```python
from build123d import *

# Parameters (mm, degrees)
SKETCH1_W           = 48.26
SKETCH1_H           = 38.1
BOSS_EXTRUDE1_DEPTH = 6.35
SKETCH2_R           = 3.683
CUT_EXTRUDE1_DEPTH  = 4.318
SKETCH3_R           = 2.159
CUT_EXTRUDE2_DEPTH  = 4.318
SKETCH4_R           = 1.143
CUT_EXTRUDE3_DEPTH  = 9.398
LPATTERN1_COUNT     = 3
LPATTERN1_PITCH     = 19.05
CUT_EXTRUDE7_DEPTH  = 4.318
CUT_EXTRUDE8_DEPTH  = 10.16


with BuildPart() as part:
    # Sketch1 → Boss-Extrude1 (new body)
    with BuildSketch(Plane(origin=(0, 0, 0), x_dir=(1, 0, 0), z_dir=(0, 1, 0))):
        Rectangle(SKETCH1_W, SKETCH1_H)
    extrude(amount=-BOSS_EXTRUDE1_DEPTH)

    # Sketch2 → Cut-Extrude1 (cut)
    with BuildSketch(Plane(origin=(0, 0, 0), x_dir=(1, 0, 0), z_dir=(0, 1, 0))):
        with Locations((-13.97, 0)):
            Circle(SKETCH2_R)
    cut_extrude1 = extrude(amount=-CUT_EXTRUDE1_DEPTH, mode=Mode.SUBTRACT)

    # Sketch3 → Cut-Extrude2 (cut)
    with BuildSketch(Plane(origin=(0, -4.318, 0), x_dir=(1, 0, 0), z_dir=(0, 1, 0))):
        with Locations((-13.97, 0)):
            Circle(SKETCH3_R)
    cut_extrude2 = extrude(amount=-CUT_EXTRUDE2_DEPTH, mode=Mode.SUBTRACT)

    # Sketch4 → Cut-Extrude3 (cut)
    with BuildSketch(Plane(origin=(0, 0, 0), x_dir=(1, 0, 0), z_dir=(0, 1, 0))):
        with Locations((-19.05, 15.621)):
            Circle(SKETCH4_R)
        with Locations((-19.05, -15.621)):
            Circle(SKETCH4_R)
    cut_extrude3 = extrude(amount=-CUT_EXTRUDE3_DEPTH, mode=Mode.SUBTRACT)

    # LPattern1: Cut-Extrude3 ×3
    with Locations(*[(i * LPATTERN1_PITCH, 0, 0) for i in range(1, LPATTERN1_COUNT)]):
        add(cut_extrude3, mode=Mode.SUBTRACT)

    # Mirror1: Cut-Extrude1, Cut-Extrude2 across plane
    add(cut_extrude1.mirror(Plane(origin=(0, 0, 0), x_dir=(0, 0, 1), z_dir=(1, 0, 0))), mode=Mode.SUBTRACT)
    add(cut_extrude2.mirror(Plane(origin=(0, 0, 0), x_dir=(0, 0, 1), z_dir=(1, 0, 0))), mode=Mode.SUBTRACT)

    # Sketch6 → Cut-Extrude7 (cut)
    with BuildSketch(Plane(origin=(0, 0, 0), x_dir=(1, 0, 0), z_dir=(0, 1, 0))):
        with BuildLine():
            Line((-17.653, -8.89), (-17.653, 8.89))
            ThreePointArc((-17.653, 8.89), (-13.97, 12.573), (-10.287, 8.89))
            Line((-10.287, 8.89), (-10.287, -8.89))
            ThreePointArc((-10.287, -8.89), (-13.97, -12.573), (-17.653, -8.89))
        make_face()
    cut_extrude7 = extrude(amount=-CUT_EXTRUDE7_DEPTH, mode=Mode.SUBTRACT)

    # Sketch7 → Cut-Extrude8 (cut)
    with BuildSketch(Plane(origin=(0, -4.318, 0), x_dir=(1, 0, 0), z_dir=(0, 1, 0))):
        with BuildLine():
            Line((-16.129, -8.89), (-16.129, 8.89))
            ThreePointArc((-16.129, 8.89), (-13.97, 11.049), (-11.811, 8.89))
            Line((-11.811, 8.89), (-11.811, -8.89))
            ThreePointArc((-11.811, -8.89), (-13.97, -11.049), (-16.129, -8.89))
        make_face()
    cut_extrude8 = extrude(amount=-CUT_EXTRUDE8_DEPTH, mode=Mode.SUBTRACT)

    # Mirror2: Cut-Extrude7, Cut-Extrude8 across plane
    add(cut_extrude7.mirror(Plane(origin=(0, 0, 0), x_dir=(0, 0, 1), z_dir=(1, 0, 0))), mode=Mode.SUBTRACT)
    add(cut_extrude8.mirror(Plane(origin=(0, 0, 0), x_dir=(0, 0, 1), z_dir=(1, 0, 0))), mode=Mode.SUBTRACT)


solid = part.part
```
Here's how the part is built. I have some questions about the finished solid (model axes, mm). A direction names the side the tool comes from. Round coordinates to 2 decimals unless told otherwise and drop trailing zeros. Loops run counter-clockwise (first coordinate to the right, second up) from the corner with the lowest first, then second, coordinate; pieces in that order, holes last.
1. Will these pins go through, and if not, where does the flat tip stop? pin 1 (1.8 mm diameter, centred on x = 0, z = 15.621, fed in from -Y); pin 2 (3.5 mm diameter, centred on x = 19.05, z = -15.621, fed in from +Y).
Answers:
pin 1: passes through
pin 2: stops at y = 0
2. Thinking about a two-plate mould opening in Z: for faces 1 (the face through (-16.129, -5, 0)), 2 (the face through (24.13, -3, 0)), 3 (the face through (0, -3, 19.05)), which applies, released by +Z, released by -Z, zero draft, split by the parting line, or undercut?
Answers:
face 1: undercut
face 2: zero draft
face 3: released by +Z
3. Suppose I cut it at A-A, the plane z = 5. Please give me the cut outline in (x, y).
Answers:
outline: (-24.13, -6.35) - (-16.13, -6.35) - (-16.13, -4.32) - (-17.65, -4.32) - (-17.65, 0) - (-24.13, 0) - close; (-11.81, -6.35) - (11.81, -6.35) - (11.81, -4.32) - (10.29, -4.32) - (10.29, 0) - (-10.29, 0) - (-10.29, -4.32) - (-11.81, -4.32) - close; (16.13, -6.35) - (24.13, -6.35) - (24.13, 0) - (17.65, 0) - (17.65, -4.32) - (16.13, -4.32) - close
4. For faces 4 (the face through (-11, -4.318, 0)), 5 (the face through (11.811, -5, 0)), 6 (the face through (-24.13, -3, 0)), which set-ups out of +Z, -Z, +X, -X, +Y, -Y let a thin tool reach every point of the face, with its end or its side?
Answers:
face 4: +Y
face 5: +Y, -Y
face 6: +Z, -Z, -X, +Y, -Y
5. Suppose I cut it at C-C, the plane x = -19.05. Please give me the cut outline in (y, z), and give its area (3 significant figures).
Answers:
outline: (-6.35, -19.05) - (0, -19.05) - (0, -16.76) - (-6.35, -16.76) - close; (-6.35, -14.48) - (0, -14.48) - (0, 14.48) - (-6.35, 14.48) - close; (-6.35, 16.76) - (0, 16.76) - (0, 19.05) - (-6.35, 19.05) - close
area: 213 mm2
6. Suppose I cut it at D-D, the plane y = -3.75. Give the number of separate pieces and of enclosed holes in the cut face, and give its area (3 significant figures).
Answers:
separate pieces: 1
enclosed holes: 8
area: 1,470 mm2
7. Suppose I cut it at B-B, the plane x = -13.97. Please give me the cut outline in (y, z).
Answers:
outline: (-6.35, -19.05) - (0, -19.05) - (0, -12.57) - (-4.32, -12.57) - (-4.32, -11.05) - (-6.35, -11.05) - close; (-6.35, 11.05) - (-4.32, 11.05) - (-4.32, 12.57) - (0, 12.57) - (0, 19.05) - (-6.35, 19.05) - close
8. If I drill on probe 1 along X at (y, z) = (-3.25, 7.5); probe 2 along X at (y, z) = (-5.25, 6); probe 3 along Z at (x, y) = (19.05, -1.5), over which ranges is the centre line in solid material (lowest first)?
Answers:
probe 1: x = -24.13 to -17.65, -10.29 to 10.29, 17.65 to 24.13
probe 2: x = -24.13 to -16.13, -11.81 to 11.81, 16.13 to 24.13
probe 3: z = -19.05 to -16.76, -14.48 to 14.48, 16.76 to 19.05
